Geometry check sheet. Reference: drawing and pictorial views, mm from the part's lowest x, y, z. Round coordinates to 2 decimals unless told otherwise and drop trailing zeros. Write each loop counter-clockwise with the first axis right and the second up, starting at its lowest first coordinate (ties: lowest second). Pieces come first, ordered by that corner, then holes.
Item 1: Depth check by flat-ended pin: pin 1 (4 mm diameter, centred on x = 12, y = 25.5, fed in from +Z). Enter the tip coordinate at first touch or a pass-through.
Item 2: Material ranges on line 1 along Z through (x, y) = (50.5, 69.5); line 2 along X through (y, z) = (70.5, 5); line 3 along Y through (x, z) = (41, 70.5), recorded low to high.
Item 3: Section check B-B, the plane x = 14.5. Record the cut outline in (y, z), plus the area to 3 significant figures.
Item 4: Section check A-A, the plane y = 57. Record the cut outline in (x, z), plus the area to 3 significant figures.
Item 5: Section check C-C, the plane z = 96. Record the cut outline in (x, y) (3 decimals), plus the area to 3 significant figures.
Item 6: Release check for a two-part mould opening along Y. For the marked faces 1, 2 and 3 record: pulls with the +Y half, pulls with the -Y half, needs draft (parallel to the pull), parting line crosses it, or undercut.
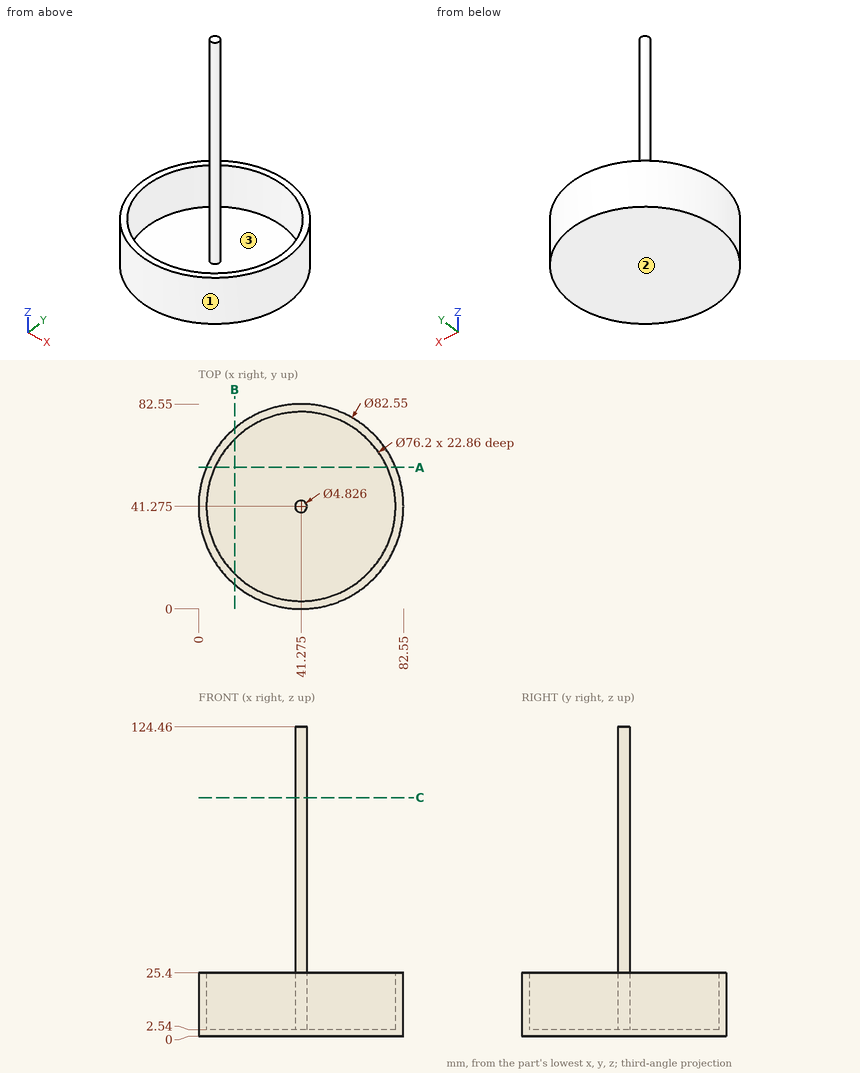
Values found:
1. pin 1: stops at z = 2.54
2. line 1: z = 0 to 2.54
2. line 2: x = 12.13 to 16.83, 65.72 to 70.42
2. line 3: y = 38.88 to 43.67
3. outline: (9.86, 0) - (72.69, 0) - (72.69, 25.4) - (68.38, 25.4) - (68.38, 2.54) - (14.17, 2.54) - (14.17, 25.4) - (9.86, 25.4) - close
3. area: 356 mm2
4. outline: (3.11, 0) - (79.44, 0) - (79.44, 25.4) - (75.98, 25.4) - (75.98, 2.54) - (6.57, 2.54) - (6.57, 25.4) - (3.11, 25.4) - close
4. area: 352 mm2
5. outline: circle Ø4.826 at (41.275, 41.275)
5. area: 18.3 mm2
6. face 1: parting line crosses it
6. face 2: needs draft
6. face 3: undercut
